from build123d import *

# Parameters (mm, degrees)
ESBO_O1_R                     = 5
RESSALTO_EXTRUS_O1_DEPTH      = 30
ESBO_O2_R                     = 4.8
CORTE_EXTRUS_O1_DEPTH         = 30
RESSALTO_EXTRUS_O2_DEPTH      = 1
RESSALTO_EXTRUS_O2_DEPTH_BACK = 1
ESBO_O3_R                     = 5.2
ESBO_O4_R                     = 3.7
RESSALTO_EXTRUS_O3_DEPTH      = 1
RESSALTO_EXTRUS_O6_DEPTH      = 1
RESSALTO_EXTRUS_O6_DEPTH_BACK = 1
ESBO_O7_R                     = 5.2
FILETE1_R                     = 0.2


with BuildPart() as part:
    # Esboço1 → Ressalto-extrusão1 (new body)
    with BuildSketch(Plane.XY):
        with Locations((-12.745849563, -1.537898167)):
            Circle(ESBO_O1_R)
    extrude(amount=RESSALTO_EXTRUS_O1_DEPTH)

    # Esboço2 → Corte-extrusão1 (cut)
    with BuildSketch(Plane.XY.offset(30)):
        with Locations((-12.745849563, -1.537898167)):
            Circle(ESBO_O2_R)
    extrude(amount=-CORTE_EXTRUS_O1_DEPTH, mode=Mode.SUBTRACT)

    # Esboço3 → Ressalto-extrusão2 (add, two sides: drawn at the far end of the back side and taken through both)
    with BuildSketch(Plane.XY.offset(30).offset(-RESSALTO_EXTRUS_O2_DEPTH_BACK)):
        with Locations((-12.745849563, -1.537898167)):
            Circle(ESBO_O3_R)
    extrude(amount=RESSALTO_EXTRUS_O2_DEPTH + RESSALTO_EXTRUS_O2_DEPTH_BACK)

    # Esboço4 → Ressalto-extrusão3 (add)
    with BuildSketch(Plane.XY.offset(31)):
        with Locations((-12.745849563, -1.537898167)):
            Circle(ESBO_O4_R)
    extrude(amount=RESSALTO_EXTRUS_O3_DEPTH)

    # Esboço7 → Ressalto-extrusão6 (add, two sides: drawn at the far end of the back side and taken through both)
    with BuildSketch(Plane(origin=(0, 0, 0), x_dir=(-1, 0, 0), z_dir=(0, 0, -1)).offset(-RESSALTO_EXTRUS_O6_DEPTH_BACK)):
        with Locations(Location((12.745849563, -1.537898167, 0), (0, 0, 180))):
            Circle(ESBO_O7_R)
    extrude(amount=RESSALTO_EXTRUS_O6_DEPTH + RESSALTO_EXTRUS_O6_DEPTH_BACK)

    # Filete1
    filete1_edges = [part.edges().sort_by_distance(p)[0] for p in [
        (-17.745849563, -1.537898167, 29),
        (-16.445849563, -1.537898167, 31),
        (-16.445849563, -1.537898167, 32),
        (-17.745849563, -1.537898167, 1),
        (-17.945849563, -1.537898167, -1),
    ]]
    fillet(filete1_edges, radius=FILETE1_R - 0.0001)  # a hair under: the kernel refuses the full size


solid = part.part
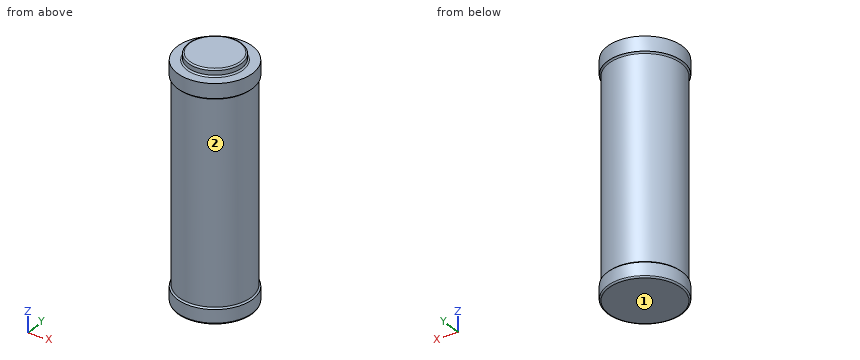
Design review of the part built by this model. Coordinates are the model's own, in mm. Face numbers are marked on the shaded views. A direction names the side the tool comes from. Coordinates: 2 decimals unless noted, no trailing zeros. Order: outer loops, then holes, each group sorted by start corner. A loop starts at its lowest first (then second) coordinate and runs counter-clockwise, first axis right, second up. Notation, with made-up numbers: (-26.5, 50) -> (-18.5, 50) arc R23 cw to (-18.5, 87) -> close; hole circle Ø4 at (32.25, 74). An arc over 180 degrees is marked (long way). Use one line per item in the form item = value. Start each with the question number.
(1) For probe 1 along Z at (x, y) = (-15.5, -5); probe 2 along X at (y, z) = (-1.5, 11.5); probe 3 along Z at (x, y) = (-13.75, -1), list the stretches that pass through material, from the lowest coordinate up.
(2) Insertion check: pin 1 (5 mm diameter, centred on y = -3, z = 24, fed in from -X); pin 2 (3 mm diameter, centred on x = -16.5, y = 0, fed in from +Z); pin 3 (6 mm diameter, centred on y = -2, z = 7.5, fed in from +X); pin 4 (3 mm diameter, centred on y = -3.5, z = 11, fed in from +X). Each pin has a flat end and moves straight along its axis. Give the tip position at first contact, or say it passes through.
(3) For the marked faces 1 and 2, list the 3-axis set-ups (+Z, -Z, +X, -X, +Y, -Y) from which the entire face can be reached by the end or side of a thin tool; tool diameter is ignored.
(4) Add section B-B on z = 30. State the section outline as (x, y) points, plus the area to 3 significant figures.
(5) Add section A-A on z = 13.5. State the section outline as (x, y) points.
Answer block:
q1.probe_1 = -1 to 1, 29 to 31
q1.probe_2 = -17.75 to -17.55, -7.95 to -7.75
q1.probe_3 = -1 to 1, 29 to 32
q2.pin_1 = -17.75
q2.pin_2 = 32
q2.pin_3 = -7.75
q2.pin_4 = -7.77
q3.face_1 = -Z, +X, -X, +Y, -Y
q3.face_2 = none
q4.outline = circle Ø10.4 at (-12.75, -1.54)
q4.area = 84.9 mm²
q5.outline = circle Ø10 at (-12.75, -1.54); hole circle Ø9.6 at (-12.75, -1.54)
